```python
from build123d import *

# Parameters (mm, degrees)
EXTRUDE_1_DEPTH     = 4
SKETCH_2_R          = 3
EXTRUDE_2_DEPTH     = 20
CUT_EXTRUDE_1_DEPTH = 1.5
CUT_EXTRUDE_2_DEPTH = 4.5
CHAMFER_2_SIZE      = 1


with BuildPart() as part:
    # Эскиз1 → Бобышка-Вытянуть1 (new body, symmetric)
    with BuildSketch(Plane.XY):
        Polygon((8.25, 0), (-8.25, 0), (-8.25, 3.5), (-4, 3.5), (-4, 5), (4, 5), (4, 3.5), (8.25, 3.5), align=None)
    extrude(amount=EXTRUDE_1_DEPTH, both=True)

    # Эскиз2 → Бобышка-Вытянуть2 (add)
    with BuildSketch(Plane(origin=(0, 5, 0), x_dir=(1, 0, 0), z_dir=(0, 1, 0))):
        with Locations(Location((0, 0, 0), (0, 0, 270))):  # turned: the seam where the file's is
            Circle(SKETCH_2_R)
    extrude(amount=EXTRUDE_2_DEPTH)

    # Эскиз3 → Вырез-Вытянуть1 (cut)
    with BuildSketch(Plane(origin=(0, 5, 0), x_dir=(1, 0, 0), z_dir=(0, 1, 0))):
        with BuildLine():
            Line((-4, 0), (-4, 4))
            Line((-4, 4), (0, 4))
            ThreePointArc((0, 4), (-2.828427125, 2.828427125), (-4, 0))
        make_face()
        with BuildLine():
            Line((0, -4), (4, -4))
            Line((4, -4), (4, 0))
            ThreePointArc((4, 0), (2.828427125, -2.828427125), (0, -4))
        make_face()
    extrude(amount=-CUT_EXTRUDE_1_DEPTH, mode=Mode.SUBTRACT)

    # Эскиз4 → Вырез-Вытянуть2 (cut, through all)
    with BuildSketch(Plane(origin=(0, 3.5, 0), x_dir=(1, 0, 0), z_dir=(0, 1, 0))):
        with BuildLine():
            Line((-7.215434845, 4), (-8.25, 4))
            Line((-8.25, 4), (-8.25, 0))
            ThreePointArc((-8.25, 0), (-7.987172136, 2.065812495), (-7.215434845, 4))
        make_face()
        with BuildLine():
            Line((7.215434845, -4), (8.25, -4))
            Line((8.25, -4), (8.25, 0))
            ThreePointArc((8.25, 0), (7.987172136, -2.065812495), (7.215434845, -4))
        make_face()
    extrude(amount=-CUT_EXTRUDE_2_DEPTH, mode=Mode.SUBTRACT)

    # Вырез-По траектории1: sweep along a path in Эскиз6
    with BuildLine(Plane.XZ) as sweep_1_path:
        Line((0, -8.25), (8.25, -8.25))
        Line((8.25, -8.25), (8.25, 0))
        ThreePointArc((8.25, 0), (5.833630945, 5.833630945), (0, 8.25))
        Line((0, 8.25), (-8.25, 8.25))
        Line((-8.25, 8.25), (-8.25, 0))
        ThreePointArc((-8.25, 0), (-5.833630945, -5.833630945), (0, -8.25))
    # Эскиз5 → Вырез-По траектории1 (sweep, cut)
    with BuildSketch(Plane.XY.offset(4)):
        Polygon((-8.25, 2), (-4.8, 0), (-8.25, 0), align=None)
    sweep(path=sweep_1_path.line, transition=Transition.RIGHT, mode=Mode.SUBTRACT)

    # Фаска2
    chamfer_2_edges = [part.edges().sort_by_distance(p)[0] for p in [
        (0, 25, -3),
    ]]
    chamfer(chamfer_2_edges, length=CHAMFER_2_SIZE)


solid = part.part
```
The model under review builds one solid part; all positions refer to its coordinate system, in mm. A direction names the side the tool comes from. Give positions to 0.01 mm unless a question says otherwise; leave off trailing zeros. Write each loop counter-clockwise with the first axis right and the second up, starting at its lowest first coordinate (ties: lowest second). Pieces come first, ordered by that corner, then holes.
(1) Consider section A-A, the plane y = 21.5. Give the boundary of the cut face in (x, z).
(2) Tool access review of faces 1 (the cylindrical face through (0.9, 14.37, 2.86)), 2 (the cylindrical face through (2.859, 4.26, 2.797)), 3 (the flat face through (-4, 4, 2)): name each direction out of +Z, -Z, +X, -X, +Y, -Y from which nothing blocks a thin tool from reaching the whole face with its end or side.
(3) To check wall thickness, follow L1, parallel to Y at x = 4.5, z = -1.75; L2, parallel to Y at x = -2.5, z = -2.5; L3, parallel to Z at x = 2.5, y = 6.5. State the ranges of each line that lie inside material, in increasing order.
(4) For P1, Ø3, axis at y = 14.5, z = -0.5, coming from the +X side; P2, Ø1, axis at y = 17.5, z = -1.5, coming from the +X side; P3, Ø5, axis at x = 2, y = 10, coming from the -Z side; P4, Ø2.5, axis at x = 3, z = 1, coming from the +Y side, all flat-tipped, find the tip position at first contact; note any pin that passes through.
Returned:
1. outline: circle Ø6 at (0, 0)
2. face 1: +Y
2. face 2: +Z, +X, +Y
2. face 3: +Z, -Z, -X, +Y
3. L1: y = 0 to 3.5
3. L2: y = 0 to 5
3. L3: z = -1.66 to 1.66
4. P1: stops at x = 3
4. P2: stops at x = 2.83
4. P3: stops at z = -3
4. P4: stops at y = 25
